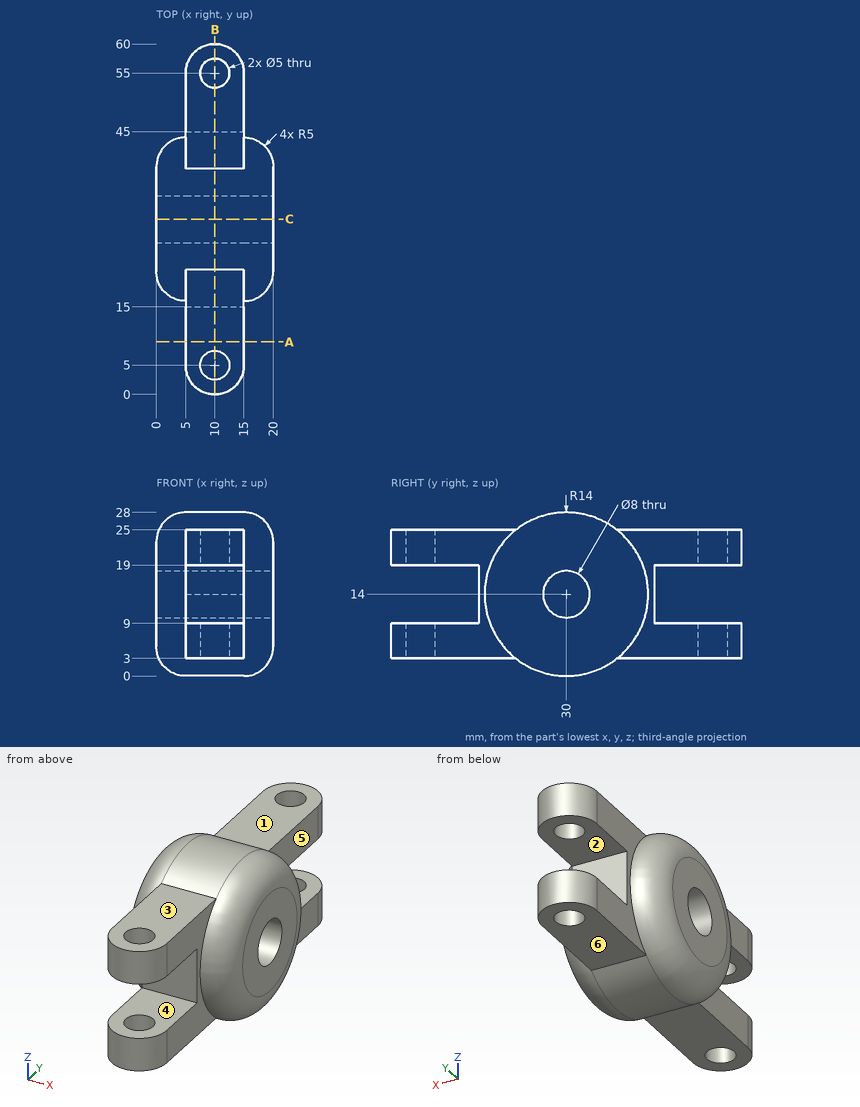
Answer from the drawing. Dimensions are ordinates in mm from the lowest x, y and z of the part. A direction names the side the tool comes from. Coordinates: 2 decimals unless noted, no trailing zeros. Order: outer loops, then holes, each group sorted by start corner. A loop starts at its lowest first (then second) coordinate and runs counter-clockwise, first axis right, second up. Notation, with made-up numbers: (40.25, -36.5) - (86.25, -36.5) arc R13 cw to (86.25, -32.5) - close; hole circle Ø4 at (89.5, -27.75). An arc over 180 degrees is marked (long way). Use one line per item in the form item = value.
(1) Straight lines are drawn through the part: L1, parallel to Y at x = 10, z = 5.5; L2, parallel to Z at x = 10.25, y = 8; L3, parallel to Y at x = 9, z = 19.5. For each, find the intervals that lie inside material, in ascending order.
Computed values:
L1 = 0 to 2.5, 7.5 to 52.5, 57.5 to 60
L2 = 3 to 9, 19 to 25
L3 = 0.1 to 2.71, 7.29 to 52.71, 57.29 to 59.9
(2) Section A-A, the plane y = 9 is taken. Give the vertices of the cut face in (x, z), then the cut area to 3 significant figures.
Computed values:
outline = (5, 3) - (15, 3) - (15, 9) - (5, 9) - close; (5, 19) - (15, 19) - (15, 25) - (5, 25) - close
area = 120 mm²
(3) Which of the six approach directions +Z, -Z, +X, -X, +Y, -Y give full straight-line access (tool end or side, diameter ignored) to the marked faces 1, 2 and 3?
Computed values:
face_1 = +Z, +X, -X, +Y
face_2 = +X, -X, +Y
face_3 = +Z, +X, -X, -Y
(4) Section C-C, the plane y = 30 is taken. Give the vertices of the cut face in (x, z), then the cut area to 3 significant figures.
Computed values:
outline = (0, 5) arc R5 ccw to (5, 0) - (15, 0) arc R5 ccw to (20, 5) - (20, 10) - (0, 10) - close; (0, 18) - (20, 18) - (20, 23) arc R5 ccw to (15, 28) - (5, 28) arc R5 ccw to (0, 23) - close
area = 379 mm²
(5) Given pin 1 Ø13 at (y, z) = (11.5, 10) entering from +X; pin 2 Ø5 at (x, y) = (11, 15) entering from +Z; pin 3 Ø12 at (x, y) = (16.5, 18) entering from +Z, each flat-ended and moving along its own axis, determine where each tip first touches the part or whether it passes through.
Computed values:
pin_1 = 18.64
pin_2 = 25
pin_3 = 26.58
(6) For a pull along Z with two mould halves and no side action, classify the marked faces 4, 5 and 6 as pulls with the +Z half, pulls with the -Z half, needs draft (parallel to the pull), parting line crosses it, or undercut.
Computed values:
face_4 = undercut
face_5 = needs draft
face_6 = pulls with the -Z half
(7) Section B-B, the plane x = 10 is taken. Give the number of separate pieces and of enclosed holes in the cut face, then the cut area to 3 significant figures.
Computed values:
separate_pieces = 5
enclosed_holes = 1
area = 921 mm²
